```python
from build123d import *

# Parameters (mm, degrees)
CROQUIS1_W                 = 45
CROQUIS1_H                 = 45
SALIENTE_EXTRUIR1_DEPTH    = 300
CROQUIS4_W                 = 18
CROQUIS4_H                 = 34
CORTAR_EXTRUIR2_DEPTH      = 46
CROQUIS8_W                 = 35
CROQUIS8_H                 = 35
CORTAR_EXTRUIR3_DEPTH      = 301
CROQUIS9_W                 = 35
CROQUIS9_H                 = 21.174410022
CORTAR_EXTRUIR4_DEPTH      = 10
CROQUIS10_R                = 1
CORTAR_EXTRUIR5_DEPTH      = 10
CROQUIS11_W                = 45
CROQUIS11_H                = 26.387879272
CORTAR_EXTRUIR6_DEPTH      = 46
CROQUIS13_W                = 45
CROQUIS13_H                = 100
CORTAR_EXTRUIR9_DEPTH      = 23.5
CORTAR_EXTRUIR9_DEPTH_BACK = 23.5
CROQUIS14_W                = 55
CROQUIS14_H                = 55
CROQUIS14_R                = 1
SALIENTE_EXTRUIR3_DEPTH    = 5


with BuildPart() as part:
    # Croquis1 → Saliente-Extruir1 (new body)
    with BuildSketch(Plane(origin=(0, 0, 0), x_dir=(1, 0, 0), z_dir=(0, 1, 0))):
        Rectangle(CROQUIS1_W, CROQUIS1_H)
    extrude(amount=SALIENTE_EXTRUIR1_DEPTH)

    # Croquis4 → Cortar-Extruir2 (cut, through all)
    with BuildSketch(Plane.ZY.offset(22.5)):
        with Locations((13.5, 17)):
            Rectangle(CROQUIS4_W, CROQUIS4_H)
    extrude(amount=-CORTAR_EXTRUIR2_DEPTH, mode=Mode.SUBTRACT)

    # Croquis8 → Cortar-Extruir3 (cut, through all)
    with BuildSketch(Plane(origin=(0, 300, 0), x_dir=(1, 0, 0), z_dir=(0, 1, 0))):
        Rectangle(CROQUIS8_W, CROQUIS8_H)
    extrude(amount=-CORTAR_EXTRUIR3_DEPTH, mode=Mode.SUBTRACT)

    # Croquis9 → Cortar-Extruir4 (cut)
    with BuildSketch(Plane(origin=(0, 0, -22.5), x_dir=(-1, 0, 0), z_dir=(0, 0, -1))):
        with Locations((0, 260)):
            Rectangle(CROQUIS9_W, CROQUIS9_H)
    extrude(amount=-CORTAR_EXTRUIR4_DEPTH, mode=Mode.SUBTRACT)

    # Croquis10 → Cortar-Extruir5 (cut)
    with BuildSketch(Plane.XY.offset(22.5)):
        with Locations((0, 260)):
            Circle(CROQUIS10_R)
    extrude(amount=-CORTAR_EXTRUIR5_DEPTH, mode=Mode.SUBTRACT)

    # Croquis11 → Cortar-Extruir6 (cut, through all)
    with BuildSketch(Plane.XY.offset(22.5)):
        with Locations((0, 286.806060364)):
            Rectangle(CROQUIS11_W, CROQUIS11_H)
    extrude(amount=-CORTAR_EXTRUIR6_DEPTH, mode=Mode.SUBTRACT)

    # Croquis13 → Cortar-Extruir9 (cut, two sides)
    with BuildSketch(Plane(origin=(0, 0, 0), x_dir=(0, 0, -1), z_dir=(1, 0, 0))) as cortar_extruir9_sk:
        with Locations((0, 223.612120728)):
            Rectangle(CROQUIS13_W, CROQUIS13_H)
    extrude(amount=CORTAR_EXTRUIR9_DEPTH, mode=Mode.SUBTRACT)
    extrude(cortar_extruir9_sk.sketch, amount=-CORTAR_EXTRUIR9_DEPTH_BACK, mode=Mode.SUBTRACT)

    # Croquis14 → Saliente-Extruir3 (add)
    with BuildSketch(Plane(origin=(0, 173.612120728, 0), x_dir=(1, 0, 0), z_dir=(0, 1, 0))):
        Rectangle(CROQUIS14_W, CROQUIS14_H)
        with Locations((-25, 25)):
            Circle(CROQUIS14_R, mode=Mode.SUBTRACT)
        with Locations((25, -25)):
            Circle(CROQUIS14_R, mode=Mode.SUBTRACT)
        with Locations((25, 25)):
            Circle(CROQUIS14_R, mode=Mode.SUBTRACT)
        with Locations((-25, -25)):
            Circle(CROQUIS14_R, mode=Mode.SUBTRACT)
    extrude(amount=SALIENTE_EXTRUIR3_DEPTH)


solid = part.part
```
Build history of the part. All positions in model axes, mm. A direction names the side the tool comes from. Round coordinates to 2 decimals unless told otherwise and drop trailing zeros. Write each loop counter-clockwise with the first axis right and the second up, starting at its lowest first coordinate (ties: lowest second). Pieces come first, ordered by that corner, then holes.
1) Band-saw the part on B-B, the plane y = 138. List the corners of the cut face in (x, z), and give its area (3 significant figures).
2) 3-axis set-ups, long thin cutter, end or side, ignore diameter. For faces 4 (the flat face through (17.5, 88, 0)), 5 (the flat face through (22.5, 86, 0)), 6 (the flat face through (0, 103, 22.5)), 7 (the flat face through (-27.5, 176, 0)), 8 (the flat face through (0, 86, -22.5)): which of +Z, -Z, +X, -X, +Y, -Y reach the whole face in a straight line?
3) Band-saw the part on C-C, the plane x = -5.5. List the corners of the cut face in (y, z), and give its area (3 significant figures).
4) Band-saw the part on D-D, the plane z = 20. List the corners of the cut face in (x, y).
5) Band-saw the part on A-A, the plane z = -2. List the corners of the cut face in (x, y).
6) Drill centre lines: probe 1 along X at (y, z) = (177, 25); probe 2 along Z at (x, y) = (15, 147). Where is each one in solid material? Low to high.
7) Mould opens along Z. For faces 1 (the flat face through (-22.5, 86, 0)), 2 (the flat face through (0, 176, 27.5)), 3 (the flat face through (0, 173.612, 0)) say: +Z half, -Z half, draft (parallel to the pull), parting line (faces both ways), or undercut.
8) Pin check, flat tips, straight feed: pin 1 (1 mm diameter, centred on x = -7.5, y = 126.5, fed in from -Z); pin 2 (13.5 mm diameter, centred on y = 83.5, z = -6.5, fed in from +X); pin 3 (10.5 mm diameter, centred on x = 7.5, y = 98, fed in from +Z). Stop position of each tip, or through.
Ans:
1. outline: (-22.5, -22.5) - (22.5, -22.5) - (22.5, 22.5) - (-22.5, 22.5) - close; hole (-17.5, -17.5) - (17.5, -17.5) - (17.5, 17.5) - (-17.5, 17.5) - close
1. area: 800 mm2
2. face 4: -Y
2. face 5: +Z, -Z, +X, -Y
2. face 6: +Z, +X, -X, -Y
2. face 7: +Z, -Z, -X, +Y, -Y
2. face 8: -Z, +X, -X, -Y
3. outline: (0, -22.5) - (173.61, -22.5) - (173.61, -27.5) - (178.61, -27.5) - (178.61, 27.5) - (173.61, 27.5) - (173.61, 22.5) - (34, 22.5) - (34, 17.5) - (173.61, 17.5) - (173.61, -17.5) - (0, -17.5) - close
3. area: 1,840 mm2
4. outline: (-27.5, 173.61) - (-22.5, 173.61) - (-22.5, 34) - (22.5, 34) - (22.5, 173.61) - (27.5, 173.61) - (27.5, 178.61) - (-27.5, 178.61) - close
5. outline: (-27.5, 173.61) - (-22.5, 173.61) - (-22.5, 0) - (-17.5, 0) - (-17.5, 173.61) - (17.5, 173.61) - (17.5, 0) - (22.5, 0) - (22.5, 173.61) - (27.5, 173.61) - (27.5, 178.61) - (-27.5, 178.61) - close
6. probe 1: x = -27.5 to -26, -24 to 24, 26 to 27.5
6. probe 2: z = -22.5 to -17.5, 17.5 to 22.5
7. face 1: draft
7. face 2: +Z half
7. face 3: undercut
8. pin 1: stops at z = -22.5
8. pin 2: stops at x = 22.5
8. pin 3: stops at z = 22.5
